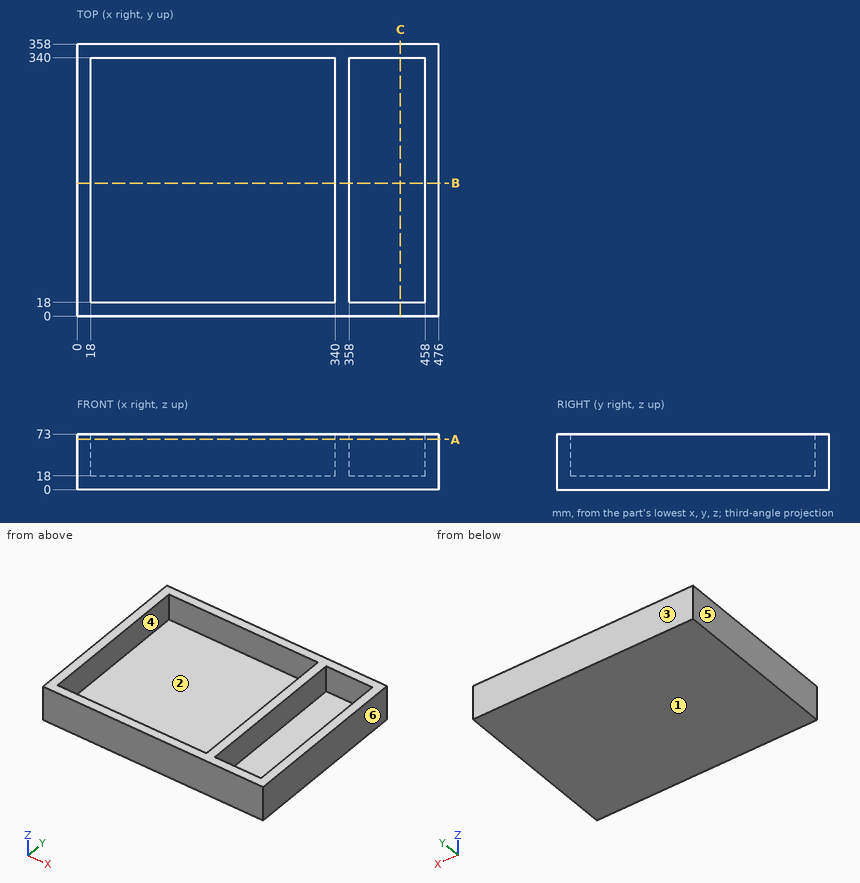
Geometry: see drawing. Coordinates: mm, zero at the bounding-box minimum. A direction names the side the tool comes from. Give positions to 0.01 mm unless a question says otherwise; leave off trailing zeros. Write each loop counter-clockwise with the first axis right and the second up, starting at its lowest first coordinate (ties: lowest second). Pieces come first, ordered by that corner, then holes. Notation, with made-up numbers: (72.25, -21.75) - (122.25, -21.75) arc R16 ccw to (122.25, -12.75) - close; hole circle Ø9 at (-30, 44). An arc over 180 degrees is marked (long way). Return JSON: item names as keys, results as strings. Group by question number.
1) First-contact query: P1, Ø8, axis at x = 159, y = 222.5, coming from the +Z side. Flat tip, straight axial feed; report the tip coordinate or a pass-through.
2) Section C-C on x = 425.5. Return the cut outline in (y, z), plus the area to 3 significant figures.
3) Section A-A on z = 66. Return the cut outline in (x, y), plus the area to 3 significant figures.
4) Line query: line 1 (X direction, y = 182.5, z = 31); line 2 (Y direction, x = 209.5, z = 38); line 3 (Z direction, x = 73.5, y = 325). Output: solid intervals per line, ascending.
5) Mould query, pull axis X, two halves, no side actions, for the marked faces 3, 4, 5 and 6. Classes: released by +X, released by -X, zero draft, split by the parting line, or undercut.
6) Section B-B on y = 175. Return the cut outline in (x, z), plus the area to 3 significant figures.
7) Set-up query: the marked faces 1 and 2. Return all of +Z, -Z, +X, -X, +Y, -Y with unobstructed straight access to the full face (end or side cutting, diameter ignored); none if empty.
Filled in:
{
 "1": {"P1": "stops at z = 18"},
 "2": {"outline": "(0, 0) - (358, 0) - (358, 73) - (340, 73) - (340, 18) - (18, 18) - (18, 73) - (0, 73) - close", "area": "8,420 mm^2"},
 "3": {"outline": "(0, 0) - (476, 0) - (476, 358) - (0, 358) - close; hole (18, 18) - (340, 18) - (340, 340) - (18, 340) - close; hole (358, 18) - (458, 18) - (458, 340) - (358, 340) - close", "area": "34,500 mm^2"},
 "4": {"line 1": "x = 0 to 18, 340 to 358, 458 to 476", "line 2": "y = 0 to 18, 340 to 358", "line 3": "z = 0 to 18"},
 "5": {"face 3": "zero draft", "face 4": "undercut", "face 5": "released by -X", "face 6": "released by +X"},
 "6": {"outline": "(0, 0) - (476, 0) - (476, 73) - (458, 73) - (458, 18) - (358, 18) - (358, 73) - (340, 73) - (340, 18) - (18, 18) - (18, 73) - (0, 73) - close", "area": "11,500 mm^2"},
 "7": {"face 1": "-Z, +X, -X, +Y, -Y", "face 2": "+Z"}
}
